Source: three-view drawing plus pictorial views. Frame: mm from the lowest corner of the part. Coordinates: 2 decimals unless noted, no trailing zeros. Order: outer loops, then holes, each group sorted by start corner. A loop starts at its lowest first (then second) coordinate and runs counter-clockwise, first axis right, second up. Notation, with made-up numbers: M 52,34 L 109,34 A20 cw 109,53 Z; hole C -16,8 d9. An arc over 180 degrees is marked long. Use CSV: the item, a comma, the result in double quotes. Start each with the question number.
Q1. Section query D-D, the plane x = 2.75. Output: boundary loops of the cut face in (y, z), and give its area (3 significant figures).
Q2. Section query A-A, the plane x = 10. Output: boundary loops of the cut face in (y, z), and give its area (3 significant figures).
Q3. Mould query, pull axis Y, two halves, no side actions, for the marked faces 1, 2, 3 and 4. Classes: +Y half, -Y half, draft (parallel to the pull), parting line (faces both ways), or undercut.
Q4. Section query B-B, the plane z = 7. Output: boundary loops of the cut face in (x, y).
Q5. Ray query, probe 1 along Y at (x, z) = (10, 7.25); probe 2 along Y at (x, z) = (8.25, 3.75); probe 3 along Y at (x, z) = (15.5, 7). Return the intervals inside material, ascending.
Q6. First-contact query: P1, Ø1, axis at x = 17.5, y = 16, coming from the -Z side; P2, Ø2.5, axis at x = 10, y = 45, coming from the -Z side. Flat tips, straight axial feed; report the tip coordinate or a pass-through.
Q7. Section query C-C, the plane y = 45. Output: boundary loops of the cut face in (x, z), and give its area (3 significant figures).
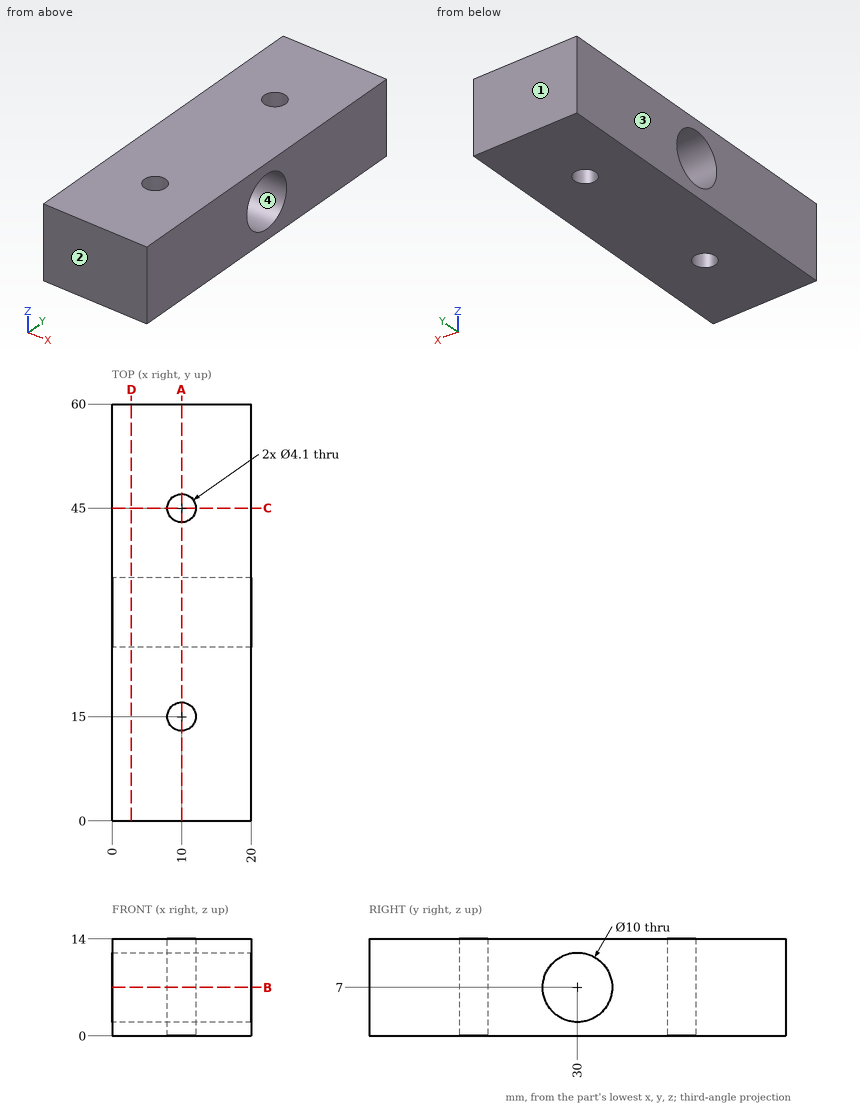
Responses:
1,outline,"M 0,0 L 60,0 L 60,14 L 0,14 Z; hole C 30,7 d10"
1,area,"761 mm²"
2,outline,"M 0,0 L 12.95,0 L 12.95,14 L 0,14 Z; M 17.05,0 L 42.95,0 L 42.95,14 L 17.05,14 Z; M 47.05,0 L 60,0 L 60,14 L 47.05,14 Z; hole C 30,7 d10"
2,area,"647 mm²"
3,face 1,"+Y half"
3,face 2,"-Y half"
3,face 3,"draft"
3,face 4,"undercut"
4,outline,"M 0,0 L 20,0 L 20,25 L 0,25 Z; M 0,35 L 20,35 L 20,60 L 0,60 Z; hole C 10,15 d4.1; hole C 10,45 d4.1"
5,probe 1,"y = 0 to 12.95, 17.05 to 25.01, 34.99 to 42.95, 47.05 to 60"
5,probe 2,"y = 0 to 13.93, 16.07 to 26.2, 33.8 to 43.93, 46.07 to 60"
5,probe 3,"y = 0 to 25, 35 to 60"
6,P1,"stops at z = 0"
6,P2,"passes through"
7,outline,"M 0,0 L 7.95,0 L 7.95,14 L 0,14 Z; M 12.05,0 L 20,0 L 20,14 L 12.05,14 Z"
7,area,"223 mm²"
